Input: part model. Units: mm. Frame: model coordinates. A direction names the side the tool comes from. Round coordinates to 2 decimals unless told otherwise and drop trailing zeros. Loops run counter-clockwise (first coordinate to the right, second up) from the corner with the lowest first, then second, coordinate; pieces in that order, holes last. Notation, with made-up numbers: (11.5, 74.25) -> (44.5, 74.25) arc R27 cw to (44.5, 101.25) -> close; hole circle Ø2 at (24.5, 63.25). An arc over 180 degrees is marked (long way). Answer as a JSON object with one key per item and string values.
```python
from build123d import *

# Parameters (mm, degrees)
SKETCH1_W                       = 110
SKETCH1_H                       = 50
BOSS_EXTRUDE1_DEPTH             = 25
SKETCH2_R                       = 7.6
CUT_EXTRUDE1_DEPTH              = 26
M8_CLEARANCE_HOLE1_D            = 10
M8_CLEARANCE_HOLE1_DEPTH        = 25
M8_CLEARANCE_HOLE1_TIP          = 3.004303095
SKETCH5_W                       = 10
SKETCH5_H                       = 50
CUT_EXTRUDE2_DEPTH              = 51
SKETCH6_W                       = 13
SKETCH6_H                       = 15
CUT_EXTRUDE3_DEPTH              = 6.8
CUT_EXTRUDE4_DEPTH              = 25
TAP_DRILL_FOR_M3X0_5_TAP1_D     = 2.5
TAP_DRILL_FOR_M3X0_5_TAP1_DEPTH = 32.5
TAP_DRILL_FOR_M3X0_5_TAP1_TIP   = 0.751075774


with BuildPart() as part:
    # Sketch1 → Boss-Extrude1 (new body)
    with BuildSketch(Plane(origin=(0, 0, 0), x_dir=(0, 0, -1), z_dir=(1, 0, 0))):
        Rectangle(SKETCH1_W, SKETCH1_H)
    extrude(amount=BOSS_EXTRUDE1_DEPTH)

    # Sketch2 → Cut-Extrude1 (cut, through all)
    with BuildSketch(Plane(origin=(25, 0, 0), x_dir=(0, 0, -1), z_dir=(1, 0, 0))):
        with Locations((-40, -0.006913882)):
            Circle(SKETCH2_R)
        with Locations((40, -0.006913882)):
            Circle(SKETCH2_R)
    extrude(amount=-CUT_EXTRUDE1_DEPTH, mode=Mode.SUBTRACT)

    # M8 Clearance Hole1
    with Locations(Plane(origin=(25, 0, 0), x_dir=(0, 0, -1), z_dir=(1, 0, 0))):
        with Locations((0, 0)):
            Hole(M8_CLEARANCE_HOLE1_D / 2, depth=M8_CLEARANCE_HOLE1_DEPTH)
            with Locations((0, 0, -(M8_CLEARANCE_HOLE1_DEPTH + M8_CLEARANCE_HOLE1_TIP / 2))):  # 118° drill point
                Cone(0, M8_CLEARANCE_HOLE1_D / 2, M8_CLEARANCE_HOLE1_TIP, mode=Mode.SUBTRACT)

    # Sketch5 → Cut-Extrude2 (cut, through all)
    with BuildSketch(Plane.XZ.offset(25)):
        with Locations((5, 0)):
            Rectangle(SKETCH5_W, SKETCH5_H)
    extrude(amount=-CUT_EXTRUDE2_DEPTH, mode=Mode.SUBTRACT)

    # Sketch6 → Cut-Extrude3 (cut)
    with BuildSketch(Plane.ZY.offset(-10)):
        Rectangle(SKETCH6_W, SKETCH6_H)
    extrude(amount=-CUT_EXTRUDE3_DEPTH, mode=Mode.SUBTRACT)

    # Sketch7 → Cut-Extrude4 (cut)
    with BuildSketch(Plane.ZY):
        with BuildLine():
            Line((-25, -25), (-25.995843668, -36.367385103))
            Line((-25.995843668, -36.367385103), (-60.780158428, -28.692554088))
            Line((-60.780158428, -28.692554088), (-59.294707264, 34.562907985))
            Line((-59.294707264, 34.562907985), (-23.260411868, 33.716701439))
            Line((-23.260411868, 33.716701439), (-25, 25))
            ThreePointArc((-25, 25), (-55, 0), (-25, -25))
        make_face()
        with BuildLine():
            Line((25, -25), (27.231233017, -36.367385103))
            Line((27.231233017, -36.367385103), (50.619615813, -36.367385103))
            Line((50.619615813, -36.367385103), (65.908125779, -26.522621757))
            Line((65.908125779, -26.522621757), (65.908125779, 30.480233283))
            Line((65.908125779, 30.480233283), (20.447589522, 40.50382591))
            Line((20.447589522, 40.50382591), (25, 25))
            ThreePointArc((25, 25), (55, 0), (25, -25))
        make_face()
    extrude(amount=-CUT_EXTRUDE4_DEPTH, mode=Mode.SUBTRACT)

    # Tap Drill for M3x0.5 Tap1
    with Locations(Plane(origin=(0, -25, 0), x_dir=(-1, 0, 0), z_dir=(0, -1, 0))):
        with Locations((-16.984771765, 19), (-16.984771765, -19)):
            Hole(TAP_DRILL_FOR_M3X0_5_TAP1_D / 2, depth=TAP_DRILL_FOR_M3X0_5_TAP1_DEPTH)
            with Locations((0, 0, -(TAP_DRILL_FOR_M3X0_5_TAP1_DEPTH + TAP_DRILL_FOR_M3X0_5_TAP1_TIP / 2))):  # 118° drill point
                Cone(0, TAP_DRILL_FOR_M3X0_5_TAP1_D / 2, TAP_DRILL_FOR_M3X0_5_TAP1_TIP, mode=Mode.SUBTRACT)


solid = part.part
```
1) Draft query along Z for faces 1 (the face through (16.78, 8.12, -18.92)), 2 (the face through (0, 6, -33)), 3 (the face through (12, 0, 55)). Return one class per face: +Z half, -Z half, draft (parallel to the pull), parting line (faces both ways), or undercut.
Output:
{"face 1": "undercut", "face 2": "draft", "face 3": "+Z half"}
2) Ray query, probe 1 along Y at (x, z) = (21.5, 0); probe 2 along X at (y, z) = (-18, 19); probe 3 along Z at (x, y) = (17.25, -20.5). Return the intervals inside material, ascending.
Output:
{"probe 1": "y = -25 to -5, 5 to 25", "probe 2": "x = 10 to 15.73, 18.23 to 25", "probe 3": "z = -44.61 to -20.22, -17.78 to 17.78, 20.22 to 44.61"}
3) Reachability of faces 4 (the face through (13, 0, -6.5)), 5 (the face through (16.71, -8.52, 20.22)), 6 (the face through (5, 0, 25)), 7 (the face through (0, 6, 34)) from +Z, -Z, +X, -X, +Y, -Y: full face, straight path, thin tool, end or side. Return the list, or none.
Output:
{"face 4": "-X", "face 5": "-Y", "face 6": "-X, +Y, -Y", "face 7": "+Z, -Z, -X, +Y, -Y"}
4) Section B-B, the plane x = 1.5. Output: boundary loops of the cut face in (y, z), plus the area to 3 significant figures.
Output:
{"outline": "(-25, -34.17) arc R25.42 ccw to (25, -34.17) -> (25, -25) -> (-25, -25) -> close; (-25, 25) -> (25, 25) -> (25, 34.17) arc R25.42 ccw to (-25, 34.17) -> close; hole circle Ø15.2 at (-0.01, -40); hole circle Ø15.2 at (-0.01, 40)", "area": "2,120 mm^2"}
5) Section D-D, the plane x = 23. Output: boundary loops of the cut face in (y, z), plus the area to 3 significant figures.
Output:
{"outline": "(-25, -34.17) arc R25.42 ccw to (25, -34.17) -> (25, 34.17) arc R25.42 ccw to (-25, 34.17) -> close; hole circle Ø15.2 at (-0.01, -40); hole circle Ø15.2 at (-0.01, 40); hole circle Ø10 at (0, 0)", "area": "4,540 mm^2"}
6) Contact query for flat-ended pins moving along their axis: P1, Ø6, axis at y = 10, z = 4.5, coming from the -X side; P2, Ø5.5, axis at x = 13, y = 3.5, coming from the +Z side; P3, Ø5.5, axis at x = 13, y = -2.5, coming from the -Z side. Output: stop coordinate, or through.
Output:
{"P1": "stops at x = 10", "P2": "stops at z = 54.99", "P3": "stops at z = -55"}
7) Section A-A, the plane y = -1. Output: boundary loops of the cut face in (x, z), plus the area to 3 significant figures.
Output:
{"outline": "(0, -54.98) -> (25, -54.98) -> (25, -47.53) -> (0, -47.53) -> close; (0, -32.47) -> (25, -32.47) -> (25, -4.9) -> (16.8, -4.9) -> (16.8, -6.5) -> (10, -6.5) -> (10, -25) -> (0, -25) -> close; (0, 25) -> (10, 25) -> (10, 6.5) -> (16.8, 6.5) -> (16.8, 4.9) -> (25, 4.9) -> (25, 32.47) -> (0, 32.47) -> close; (0, 47.53) -> (25, 47.53) -> (25, 54.98) -> (0, 54.98) -> close; hole circle Ø2.5 at (16.98, -19); hole circle Ø2.5 at (16.98, 19)", "area": "1,320 mm^2"}
8) Section C-C, the plane z = -46. Output: boundary loops of the cut face in (x, y), plus the area to 3 significant figures.
Output:
{"outline": "(0, -19.4) -> (25, -19.4) -> (25, -4.67) -> (0, -4.67) -> close; (0, 4.66) -> (25, 4.66) -> (25, 19.4) -> (0, 19.4) -> close", "area": "737 mm^2"}
